Autodesk Inventor part; units mm, degrees
ref_plane "YZ Plane" through (0, 0, 0) normal (1, 0, 0) x (0, 1, 0)
ref_plane "XZ Plane" through (0, 0, 0) normal (0, 1, 0) x (-1, 0, 0)
ref_plane "XY Plane" through (0, 0, 0) normal (0, 0, 1) x (1, 0, 0)
sketch "Sketch1" plane through (0, 0, 0) normal (0, 0, 1) x (1, 0, 0)
  line L0 (-5.7054, 0) -> (133.9946, 0)
  line L1 (133.9946, 0) -> (133.9946, 81.28)
  line L2 (133.9946, 81.28) -> (79.002, 113.03)
  line L3 (-5.7054, 0) -> (-5.7054, 78.74)
  line L4 (-5.7054, 78.74) -> (79.002, 113.03)
  point P0 (0, 0)
  dimension "d0" = 139.7
  dimension "d1" = 81.28
  dimension "d2" = 63.5
  dimension "d3" = 120
  dimension "d4" = 78.74
extrude "Extrusion1" add sketch "Sketch1" along normal blind 19.05
properties part number "side battery"
Here's how the part is built. I have some questions about the finished solid (model axes, mm). Give positions to 0.01 mm unless a question says otherwise; leave off trailing zeros. Loops run counter-clockwise (first coordinate to the right, second up) from the corner with the lowest first, then second, coordinate; pieces in that order, holes last. Notation, with made-up numbers: M 11.5,-23.75 L 28.5,-23.75 A13 cw 28.5,-2.75 Z; hole C -37,0 d3. An arc over 180 degrees is marked long. Put each result on its own line as item: value. Start each with the question number.
(1) I need wall thicknesses on line 1 along X through (y, z) = (90, 17.5); line 2 along Y through (x, z) = (36.5, 4); line 3 along Y through (x, z) = (59, 17). Which ranges of each line are inside material? Lowest first, please. Write a range as [from, to].
(2) I want a section at C-C on y = 92.5. Please give me the cut outline in (x, z).
(3) I want a section at B-B on x = 110.5. Please give me the cut outline in (y, z), then the cut area to 3 significant figures.
(4) I want a section at A-A on z = 15.5. Please give me the cut outline in (x, y), then the cut area to 3 significant figures.
(5) Will these pins go through, and if not, where does the flat tip stop? pin 1 Ø1.5 at (y, z) = (97.5, 12) entering from -X; pin 2 Ø1.5 at (x, z) = (55, 12) entering from +Y; pin 3 Ø2 at (x, z) = (111.5, 6.5) entering from -Y; pin 4 Ø8 at (x, z) = (113.5, 10) entering from +Y.
Answer block:
1. line 1: [22.11, 118.89]
1. line 2: [0, 95.82]
1. line 3: [0, 104.93]
2. outline: M 28.29,0 L 114.56,0 L 114.56,19.05 L 28.29,19.05 Z
3. outline: M 0,0 L 94.84,0 L 94.84,19.05 L 0,19.05 Z
3. area: 1,810 mm^2
4. outline: M -5.71,0 L 133.99,0 L 133.99,81.28 L 79,113.03 L -5.71,78.74 Z
4. area: 13,500 mm^2
5. pin 1: x = 38.79
5. pin 2: y = 103.62
5. pin 3: y = 0
5. pin 4: y = 95.42
